```python
from build123d import *

# Parameters (mm, degrees)
F0_W     = 12
F0_H     = 4.1
F1_DEPTH = 7
F0_H_2   = 13.95
F0_R     = 0.9
F0_R_2   = 4
F0_H_3   = 3.95
F0_R_3   = 2.5
F2_DEPTH = 2
F4_R     = 0.85
F5_DEPTH = 5


# Not quite as in the source:
# - a feature of the source that left no trace in its solid (it failed there, or was rolled back) is left out


with BuildPart() as f1:
    # F0 (on Top) → F1 (new body)
    with BuildSketch(Plane.XY):
        with Locations((-0.3663106412, 0)):
            Rectangle(F0_W, F0_H)
    extrude(amount=F1_DEPTH)

    # F0 (on Top) → F2 (join)
    with BuildSketch(Plane.XY):
        with Locations((-0.3663106412, 9.025)):
            Rectangle(F0_W, F0_H_2)
        with Locations((-0.3663106412, 3)):
            Circle(F0_R, mode=Mode.SUBTRACT)
        with Locations((-0.3663106412, 10)):
            Circle(F0_R_2, mode=Mode.SUBTRACT)
        with Locations((-0.3663106412, -4.025)):
            Rectangle(F0_W, F0_H_3)
        with Locations((-0.3663106412, -3)):
            Circle(F0_R, mode=Mode.SUBTRACT)
        with Locations((-0.3663106412, 10)):
            Circle(F0_R_2)
        with Locations((-0.3663106412, 10)):
            Circle(F0_R_3, mode=Mode.SUBTRACT)
    extrude(amount=F2_DEPTH)

    # F4 (on face) → F5 (cut)
    with BuildSketch(Plane(origin=(0, 2.05, 0), x_dir=(-1, 0, 0), z_dir=(0, 1, 0))):
        with Locations((0.3663106412, 4.45)):
            Circle(F4_R)
    extrude(amount=-F5_DEPTH, mode=Mode.SUBTRACT)


solid = f1.part
```
Check sheet for the modelled part. Datum: model origin and axes. Units: mm. A direction names the side the tool comes from. Coordinates: 2 decimals unless noted, no trailing zeros. Loops run counter-clockwise (first coordinate to the right, second up) from the corner with the lowest first, then second, coordinate; pieces in that order, holes last. Notation, with made-up numbers: M 45,40.5 L 79,40.5 A24 ccw 79,59.5 Z; hole C 68.25,72 d8. An arc over 180 degrees is marked long. Answer as a JSON object with one key per item and string values.
1. Sectioned sample at A-A on y = 3. Record the cut outline in (x, z), and give its area (3 significant figures).
Outcome:
{"outline": "M -6.37,0 L -1.27,0 L -1.27,2 L -6.37,2 Z; M 0.53,0 L 5.63,0 L 5.63,2 L 0.53,2 Z", "area": "20.4 mm²"}
2. Sectioned sample at C-C on y = 0.75. Record the cut outline in (x, z), and give its area (3 significant figures).
Outcome:
{"outline": "M -6.37,0 L 5.63,0 L 5.63,7 L -6.37,7 Z; hole C -0.37,4.45 d1.7", "area": "81.7 mm²"}
3. Access from +Z, -Z, +X, -X, +Y, -Y to the whole of each face (thin tool, end or side, straight path). Record for faces 1 (the flat face through (0, 2.05, 6)), 2 (the flat face through (0, -2.05, 6)), 3 (the flat face through (5.634, 5, 1)).
Outcome:
{"face 1": "+Z, +X, -X, +Y", "face 2": "+Z, +X, -X, -Y", "face 3": "+Z, -Z, +X, +Y, -Y"}
4. Scan lines: L1, parallel to Y at x = 0.25, z = 1; L2, parallel to Z at x = -5.5, y = 7.25; L3, parallel to Y at x = -0.25, z = 1.5. Record each from-to range of solid material in increasing order. Write a range as from..to.
Outcome:
{"L1": "-6..-3.66, -2.34..2.34, 3.66..7.58, 12.42..16", "L2": "0..2", "L3": "-6..-3.89, -2.11..2.11, 3.89..7.5, 12.5..16"}
5. Release check for a two-part mould opening along Y. For faces 4 (the flat face through (0, -6, 1)), 5 (the flat face through (0, 16, 1)), 6 (the cylindrical face through (-0.91, 7.56, 0.99)) record: pulls with the +Y half, pulls with the -Y half, needs draft (parallel to the pull), parting line crosses it, or undercut.
Outcome:
{"face 4": "pulls with the -Y half", "face 5": "pulls with the +Y half", "face 6": "undercut"}
6. Depth check by flat-ended pin: P1, Ø1.2, axis at x = 0.5, y = -5, coming from the +Z side. Enter the tip coordinate at first touch or a pass-through.
Outcome:
{"P1": "z = 2"}
7. Sectioned sample at B-B on z = 0.5. Record the cut outline in (x, y), and give its area (3 significant figures).
Outcome:
{"outline": "M -6.37,-6 L 5.63,-6 L 5.63,16 L -6.37,16 Z; hole C -0.37,10 d5; hole C -0.37,-3 d1.8; hole C -0.37,3 d1.8", "area": "239 mm²"}
8. Sectioned sample at D-D on z = 4.45. Record the cut outline in (x, y), and give its area (3 significant figures).
Outcome:
{"outline": "M -6.37,-2.05 L -1.22,-2.05 L -1.22,2.05 L -6.37,2.05 Z; M 0.48,-2.05 L 5.63,-2.05 L 5.63,2.05 L 0.48,2.05 Z", "area": "42.2 mm²"}
